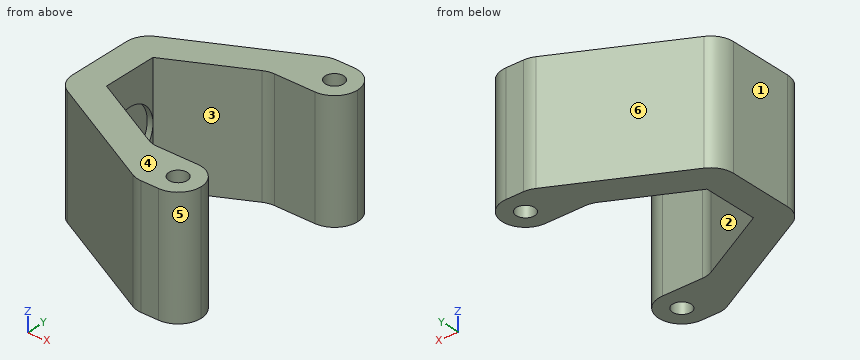
from build123d import *

# Parameters (mm, degrees)
SKETCH_R     = 1.6
PAD_DEPTH    = 20.5
SKETCH001_R  = 4.75
POCKET_DEPTH = 1
FILLET_R     = 4
FILLET001_R  = 3.9999


with BuildPart() as part:
    # Sketch → Pad (new body)
    with BuildSketch(Plane.XY):
        Polygon((18, 20), (26, 20), (26, 12), (18, 12), (14, 12), (0, 4.75), (0, -4.75), (14, -12), (18, -12), (26, -12), (26, -20), (18, -20), (-5.264538, -7.952293), (-5.264538, 7.952293), align=None)
        with Locations((22, 16)):
            Circle(SKETCH_R, mode=Mode.SUBTRACT)
        with Locations((22, -16)):
            Circle(SKETCH_R, mode=Mode.SUBTRACT)
    extrude(amount=PAD_DEPTH)

    # Sketch001 → Pocket (cut)
    with BuildSketch(Plane.YZ):
        with Locations((0, 10.25)):
            Circle(SKETCH001_R)
    extrude(amount=-POCKET_DEPTH, mode=Mode.SUBTRACT)

    # Fillet
    fillet_edges = [part.edges().sort_by_distance(p)[0] for p in [
        (26, -20, 10.25),
        (18, -20, 10.25),
        (-5.264538, -7.952293, 10.25),
        (-5.264538, 7.952293, 10.25),
        (18, 20, 10.25),
        (26, 20, 10.25),
    ]]
    fillet(fillet_edges, radius=FILLET_R)

    # Fillet001
    fillet001_edges = [part.edges().sort_by_distance(p)[0] for p in [
        (26, -12, 10.25),
        (14, -12, 10.25),
        (14, 12, 10.25),
        (26, 12, 10.25),
    ]]
    fillet(fillet001_edges, radius=FILLET001_R)


solid = part.part
Geometry: final body of the model. Coordinates: model frame, mm. Face numbers are marked on the shaded views. A direction names the side the tool comes from. Coordinates: 2 decimals unless noted, no trailing zeros. Loops run counter-clockwise (first coordinate to the right, second up) from the corner with the lowest first, then second, coordinate; pieces in that order, holes last. Notation, with made-up numbers: (-31, 41.25) - (-18, 41.25) arc R13 cw to (-18, 47.25) - close; hole circle Ø9 at (1.25, -5). An arc over 180 degrees is marked (long way). Put each result on its own line as item: value. Start each with the question number.
Q1. Cut plane D-D, the plane y = 0. Return loops of the section in (x, z), and give its area (3 significant figures).
Q2. Cut plane A-A, the plane x = 19.5. Return loops of the section in (y, z), and give its area (3 significant figures).
Q3. Line query: line 1 (Y direction, x = 22, z = 6); line 2 (Y direction, x = 23, z = 14.5); line 3 (X direction, y = 0.5, z = 14.5). Output: solid intervals per line, ascending.
Q4. Cut plane B-B, the plane z = 17.5. Give the number of separate pieces and of enclosed holes in the cut face, and give its area (3 significant figures).
Q5. Pin query (flat end, axial travel): pin 1 Ø6 at (x, y) = (-1, -16) entering from -Z; pin 2 Ø7.5 at (y, z) = (-0.5, 12.5) entering from +X; pin 3 Ø10.5 at (y, z) = (2.5, 4) entering from +X; pin 4 Ø5.5 at (y, z) = (0, 10.25) entering from +X. Return the tip coordinate at first contact, or that it passes through.
Q6. Set-up query: the marked faces 1 and 2. Return all of +Z, -Z, +X, -X, +Y, -Y with unobstructed straight access to the full face (end or side cutting, diameter ignored); none if empty.
Q7. Pull-direction query (Y, two-part tool) for the marked faces 3, 4, 5 and 6; classes: released by +Y, released by -Y, zero draft, split by the parting line, or undercut.
Q8. Cut plane C-C, the plane y = -15.5. Return loops of the section in (x, z).
Filled sheet:
1. outline: (-5.26, 0) - (0, 0) - (0, 5.5) - (-1, 5.5) - (-1, 15) - (0, 15) - (0, 20.5) - (-5.26, 20.5) - close
1. area: 98.4 mm²
2. outline: (-20, 0) - (-12, 0) - (-12, 20.5) - (-20, 20.5) - close; (12, 0) - (20, 0) - (20, 20.5) - (12, 20.5) - close
2. area: 328 mm²
3. line 1: -20 to -17.6, -14.4 to -12, 12 to 14.4, 17.6 to 20
3. line 2: -19.87 to -17.25, -14.75 to -12.13, 12.13 to 14.75, 17.25 to 19.87
3. line 3: -5.26 to -1
4. separate pieces: 1
4. enclosed holes: 2
4. area: 416 mm²
5. pin 1: through
5. pin 2: x = 0
5. pin 3: x = 5.79
5. pin 4: x = -1
6. face 1: +Z, -Z, -X, +Y, -Y
6. face 2: +Z, -Z, +X
7. face 3: undercut
7. face 4: zero draft
7. face 5: released by -Y
7. face 6: released by +Y
8. outline: (9.31, 0) - (20.48, 0) - (20.48, 20.5) - (9.31, 20.5) - close; (23.52, 0) - (25.97, 0) - (25.97, 20.5) - (23.52, 20.5) - close
